Work out the finished part from the listing and answer in its coordinate system (mm). Give positions to 0.01 mm unless a question says otherwise; leave off trailing zeros. Loops run counter-clockwise (first coordinate to the right, second up) from the corner with the lowest first, then second, coordinate; pieces in that order, holes last. Notation, with made-up numbers: M 1,26 L 44,26 A21 ccw 44,38 Z; hole C 81.25,72.5 d5. An arc over 180 degrees is marked long. Answer in a Markdown table with one row per item. Add a question column.
from build123d import *

# Parameters (mm, degrees)
F1_DEPTH = 5.08
F2_R     = 5.07999


# Not quite as in the source:
# - a fillet or chamfer is up to 0.001 mm smaller than in the source, because OpenCascade refuses the exact size


with BuildPart() as f1:
    # F0 (on Front) → F1 (new body)
    with BuildSketch(Plane.XZ):
        with BuildLine():
            Line((76.3972327113, 76.3972327113), (39.6787461365, 76.3972327113))
            ThreePointArc((39.6787461365, 76.3972327113), (3.7253e-06, 36.7184903001), (-39.678738686, 76.3972327113))
            Line((-39.678738686, 76.3972327113), (-76.3972252607, 76.3972327113))
            Line((-76.3972252607, 76.3972327113), (-76.3972252607, -115.6601980329))
            Line((-76.3972252607, -115.6601980329), (76.3972327113, -115.6601980329))
            Line((76.3972327113, -115.6601980329), (76.3972327113, 76.3972327113))
        make_face()
    extrude(amount=F1_DEPTH)

    # F2 (radius 5.08 in the source; OpenCascade refuses exactly that, so slightly less here)
    f2_edges = [f1.edges().sort_by_distance(p)[0] for p in [
        (-58.037982, -5.08, 76.397233),
        (-76.397225, -5.08, -19.631483),
        (4e-06, -5.08, 36.71849),
        (58.037989, -5.08, 76.397233),
        (76.397233, -5.08, -19.631483),
        (4e-06, -5.08, -115.660198),
    ]]
    fillet(f2_edges, radius=F2_R)


solid = f1.part
(1) Each of these flat-tipped pins is pushed along its axis until it touches: P1, Ø3, axis at x = 27, y = -4, coming from the +Z side; P2, Ø2, axis at y = -3.5, z = -92.5, coming from the -X side; P3, Ø1, axis at x = -51.5, y = -2.5, coming from the +Z side. Where does it stop, or does it pass through?
(2) Section A-A, the plane y = -2.3 is taken. Determine the outline of the cut face in (x, z), and give its area (3 significant figures).
(3) Consider line 1 along X through (y, z) = (-3.15, 64); line 2 along Z through (x, y) = (55, -1.3); line 3 along Z through (x, y) = (-13.5, -1.15). Determine where each line is inside the solid, lowest interval first. Write a range as from..to.
Numbers:
| question | item | result |
|---|---|---|
| 1 | P1 | stops at z = 47.03 |
| 1 | P2 | stops at x = -75.74 |
| 1 | P3 | stops at z = 75.99 |
| 2 | outline | M -75.85,-115.11 L 75.85,-115.11 L 75.85,75.85 L 40.23,75.85 A40.23 cw -40.23,75.85 L -75.85,75.85 Z |
| 2 | area | 26,500 mm² |
| 3 | line 1 | x = -75.3..-38.84, 38.84..75.3 |
| 3 | line 2 | z = -115.49..76.23 |
| 3 | line 3 | z = -115.53..38.95 |
